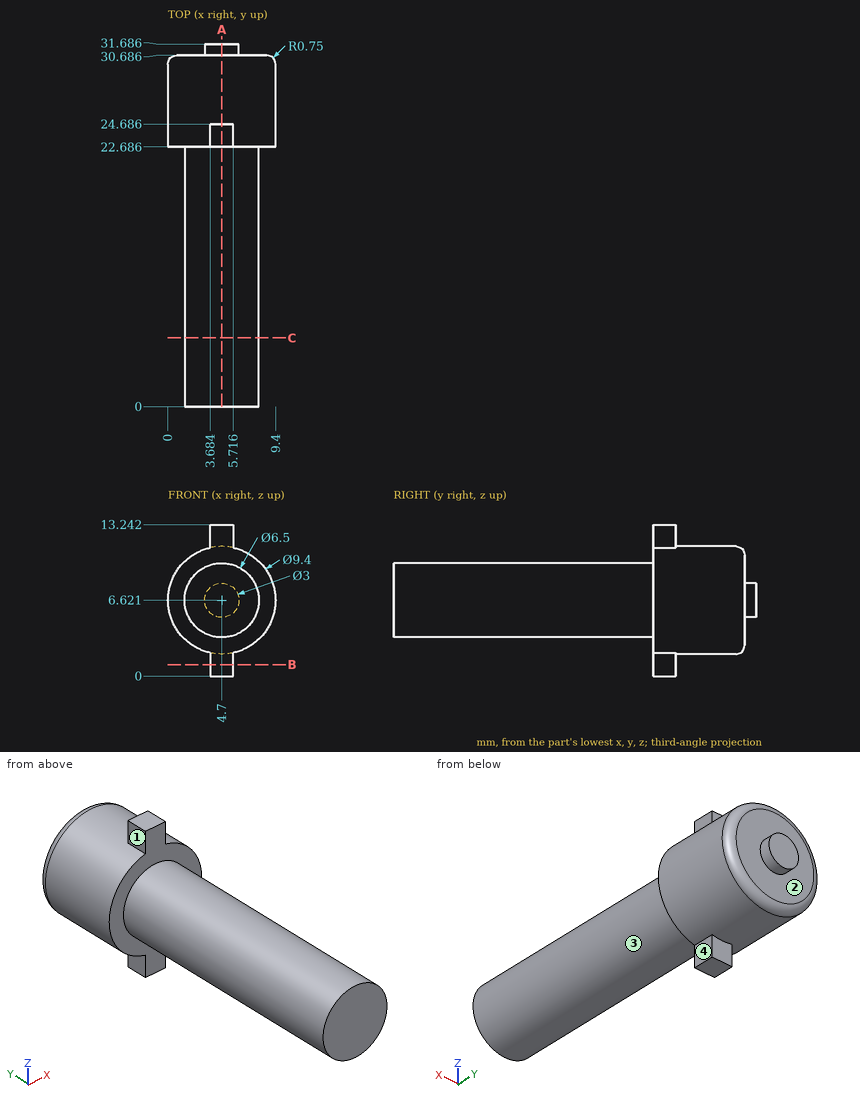
Geometry: see drawing. Coordinates: mm, zero at the bounding-box minimum. A direction names the side the tool comes from. Round coordinates to 2 decimals unless told otherwise and drop trailing zeros. Loops run counter-clockwise (first coordinate to the right, second up) from the corner with the lowest first, then second, coordinate; pieces in that order, holes last. Notation, with made-up numbers: (51, 41) -> (68, 41) arc R21 ccw to (68, 46) -> close; hole circle Ø9 at (-31.75, 68.5). An arc over 180 degrees is marked (long way). One line per question, with ' | ' between items. Start each with the question number.
1. Section C-C on y = 6. Output: boundary loops of the cut face in (x, z).
2. Set-up query: the marked faces 1, 2, 3 and 4. Return all of +Z, -Z, +X, -X, +Y, -Y with unobstructed straight access to the full face (end or side cutting, diameter ignored); none if empty.
3. Section A-A on x = 4.7. Output: boundary loops of the cut face in (y, z), and give its area (3 significant figures).
4. Line query: line 1 along Y through (x, z) = (8.5, 7.75); line 2 along Z through (x, y) = (4.75, 18); line 3 along Y through (x, z) = (2.25, 5.5). Output: solid intervals per line, ascending. Write a range as [from, to].
5. Contact query for flat-ended pins moving along their axis: pin 1 (5 mm diameter, centred on x = 6, y = 19, fed in from -Z); pin 2 (0.6 mm diameter, centred on x = 4.5, z = 1, fed in from +Y); pin 3 (2.5 mm diameter, centred on x = 5, z = 8.5, fed in from +Y); pin 4 (5 mm diameter, centred on x = 2.5, z = 2, fed in from +Y). Output: stop coordinate, or through.
6. Section B-B on z = 1. Output: boundary loops of the cut face in (x, y).
Returned:
1) outline: circle Ø6.5 at (4.7, 6.62)
2) face 1: +Z, -X, +Y, -Y | face 2: +Y | face 3: -Y | face 4: -Z, +X, +Y, -Y
3) outline: (0, 3.37) -> (22.69, 3.37) -> (22.69, 0) -> (24.69, 0) -> (24.69, 1.92) -> (29.94, 1.92) arc R0.75 ccw to (30.69, 2.67) -> (30.69, 5.12) -> (31.69, 5.12) -> (31.69, 8.12) -> (30.69, 8.12) -> (30.69, 10.57) arc R0.75 ccw to (29.94, 11.32) -> (24.69, 11.32) -> (24.69, 13.24) -> (22.69, 13.24) -> (22.69, 9.87) -> (0, 9.87) -> close | area: 233 mm2
4) line 1: y = [22.69, 30.69] | line 2: z = [3.37, 9.87] | line 3: y = [0, 30.69]
5) pin 1: stops at z = 3.37 | pin 2: stops at y = 24.69 | pin 3: stops at y = 31.69 | pin 4: stops at y = 30.69
6) outline: (3.68, 22.69) -> (5.72, 22.69) -> (5.72, 24.69) -> (3.68, 24.69) -> close
